Build history of the part. All positions in model axes, mm. Round coordinates to 2 decimals unless told otherwise and drop trailing zeros. Write each loop counter-clockwise with the first axis right and the second up, starting at its lowest first coordinate (ties: lowest second). Pieces come first, ordered by that corner, then holes. Notation, with made-up numbers: (62.5, 19.5) - (105.5, 19.5) arc R17 cw to (105.5, 49.5) - close; hole circle Ø9 at (73.5, 66.25). An arc over 180 degrees is marked (long way). One line per question, with ' | ' between items.
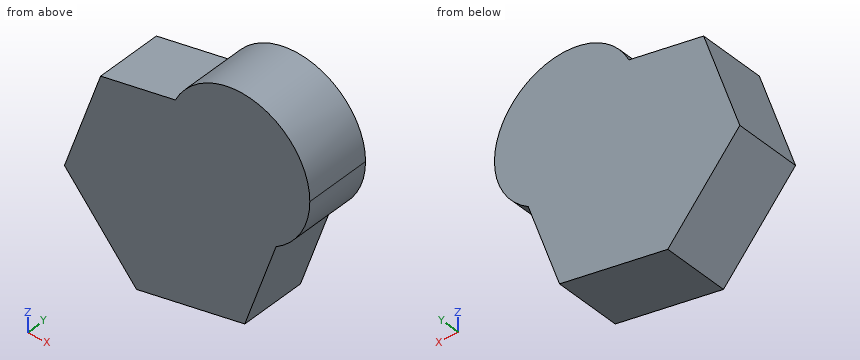
from build123d import *

# Parameters (mm, degrees)
F1_DEPTH = 50.4742488265


with BuildPart() as f1:
    # F0 (on Front) → F1 (new body)
    with BuildSketch(Plane.XZ):
        with BuildLine():
            ThreePointArc((28.4085404041, -30.6041326868), (47.4457170487, -10.8078252685), (54.3811030527, 15.7667547464))
            ThreePointArc((54.3811030527, 15.7667547464), (12.1282693342, 68.7781634448), (-48.9713224935, 39.4123450854))
            Line((-48.9713224934, 39.4123450854), (-23.2140926992, 44.3395745417))
            Line((-23.2140926992, 44.3395745417), (32.1769656266, -19.7646844725))
            Line((32.1769656266, -19.7646844725), (28.4085404041, -30.6041326868))
        make_face()
        with BuildLine():
            Line((-23.2140926992, 44.3395745417), (-48.9713224934, 39.4123450854))
            ThreePointArc((-48.9713224935, 39.4123450854), (-36.4867618694, -24.5571907142), (28.4085404041, -30.6041326868))
            Line((28.4085404041, -30.6041326868), (32.1769656266, -19.7646844725))
            Line((32.1769656266, -19.7646844725), (-23.2140926992, 44.3395745417))
        make_face()
        with BuildLine():
            ThreePointArc((28.4085404041, -30.6041326868), (-36.4867618694, -24.5571907142), (-48.9713224935, 39.4123450854))
            Line((-48.9713224934, 39.4123450854), (-106.4255386591, 28.4216403961))
            Line((-106.4255386591, 28.4216403961), (-134.2459262932, -51.6005527636))
            Line((-134.2459262932, -51.6005527636), (-78.8548679675, -115.7048117777))
            Line((-78.8548679675, -115.7048117777), (4.3565779924, -99.7868776321))
            Line((4.3565779924, -99.7868776321), (28.4085404041, -30.6041326868))
        make_face()
    extrude(amount=F1_DEPTH)


solid = f1.part
Q1. Saw through at A-A, the plane y = -15.5. List the corners of the cut face in (x, z).
Found:
outline: (-134.25, -51.6) - (-78.85, -115.7) - (4.36, -99.79) - (28.41, -30.6) arc R54.38 ccw (long way) to (-48.97, 39.41) - (-106.43, 28.42) - close
Q2. Drop flat-ended pins along their axis: pin 1 (2 mm diameter, centred on x = -21.5, y = -28, fed in from +Z); pin 2 (5 mm diameter, centred on x = -34, y = -14, fed in from +Z); pin 3 (8 mm diameter, centred on x = -90, y = -14, fed in from +Z). Give the stop position or say it passes through.
Found:
pin 1: z = 66.14 | pin 2: z = 60.1 | pin 3: z = 32.33
Q3. Saw through at B-B, the plane z = 7.5. List the corners of the cut face in (x, y), then the cut area to 3 significant figures.
Found:
outline: (-113.7, -50.47) - (53.75, -50.47) - (53.75, 0) - (-113.7, 0) - close | area: 8,450 mm^2
Q4. Drill centre lines: L1, parallel to Z at x = -53, y = -43.5; L2, parallel to Z at x = -5, y = -11.5; L3, parallel to X at y = -23.5, z = -45.5. Where is each one in solid material? Low to high. Write a range as from..to.
Found:
L1: -110.76..38.64 | L2: -101.58..69.92 | L3: -132.13..23.23
Q5. Saw through at C-C, the plane x = -42.5. List the corners of the cut face in (y, z).
Found:
outline: (-50.47, -108.75) - (0, -108.75) - (0, 49.69) - (-50.47, 49.69) - close
